The model under review builds one solid part; all positions refer to its coordinate system, in mm. Face numbers are marked on the shaded views. A direction names the side the tool comes from. Round coordinates to 2 decimals unless told otherwise and drop trailing zeros. Loops run counter-clockwise (first coordinate to the right, second up) from the corner with the lowest first, then second, coordinate; pieces in that order, holes last. Notation, with made-up numbers: (9.25, 53) -> (30.25, 53) arc R17 ccw to (30.25, 81) -> close; hole circle Ø8 at (51, 62.5). An arc over 180 degrees is marked (long way). Use CSV: the item, a comma, the result in double quotes. Start each with the question number.
```python
from build123d import *

# Parameters (mm, degrees)
SKETCH1_W           = 600
SKETCH1_H           = 310
BOSS_EXTRUDE1_DEPTH = 50
SKETCH2_W           = 515
SKETCH2_H           = 270
BOSS_EXTRUDE2_DEPTH = 160
SKETCH3_R           = 75
BOSS_EXTRUDE3_DEPTH = 26
SKETCH4_W           = 30
SKETCH4_H           = 12
BOSS_EXTRUDE4_DEPTH = 50


with BuildPart() as part:
    # Sketch1 → Boss-Extrude1 (new body)
    with BuildSketch(Plane(origin=(0, 0, 0), x_dir=(1, 0, 0), z_dir=(0, 1, 0))):
        Rectangle(SKETCH1_W, SKETCH1_H)
    extrude(amount=BOSS_EXTRUDE1_DEPTH)

    # Sketch2 → Boss-Extrude2 (add)
    with BuildSketch(Plane(origin=(0, 50, 0), x_dir=(1, 0, 0), z_dir=(0, 1, 0))):
        with Locations((0, 20)):
            Rectangle(SKETCH2_W, SKETCH2_H)
    extrude(amount=BOSS_EXTRUDE2_DEPTH)

    # Sketch3 → Boss-Extrude3 (add)
    with BuildSketch(Plane(origin=(0, 210, 0), x_dir=(1, 0, 0), z_dir=(0, 1, 0))):
        with Locations((0, 65)):
            Circle(SKETCH3_R)
    extrude(amount=BOSS_EXTRUDE3_DEPTH)

    # Sketch4 → Boss-Extrude4 (add)
    with BuildSketch(Plane(origin=(147.5, 0, 0), x_dir=(0, 0, -1), z_dir=(1, 0, 0))):
        with Locations((-65, 216)):
            Rectangle(SKETCH4_W, SKETCH4_H)
    extrude(amount=-BOSS_EXTRUDE4_DEPTH)


solid = part.part
```
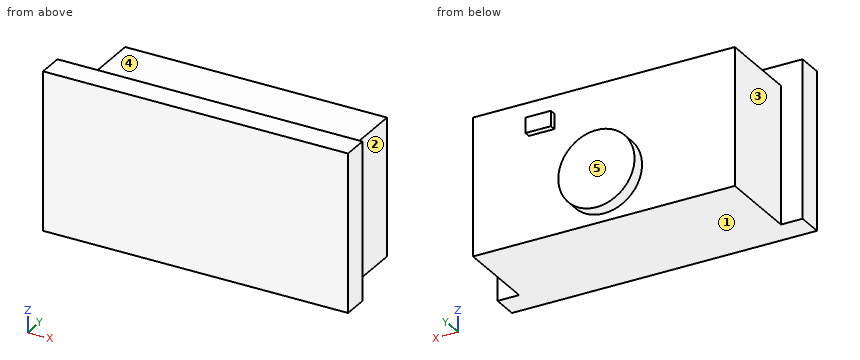
1. For the marked faces 1, 2, 3, 4 and 5, list the 3-axis set-ups (+Z, -Z, +X, -X, +Y, -Y) from which the entire face can be reached by the end or side of a thin tool; tool diameter is ignored.
2. Take a section at B-B, the plane x = 0. Give the boundary of the cut face in (y, z), then the cut area to 3 significant figures.
3. Clearance check with flat-ended pins moving along their axes: P1, Ø9.5, axis at y = 214.5, z = 65.5, coming from the +X side; P2, Ø13, axis at y = 215.5, z = 61.5, coming from the -X side; P3, Ø9.5, axis at x = 126, y = 215.5, coming from the +Z side. State where each tip first meets the part, or that it passes through.
4. Take a section at A-A, the plane z = 100. Give the boundary of the cut face in (x, y).
5. Take a section at D-D, the plane z = -65. Give the boundary of the cut face in (x, y), then the cut area to 3 significant figures.
6. Take a section at C-C, the plane y = 98. Give the boundary of the cut face in (x, z), then the cut area to 3 significant figures.
7. For line 1 along Y through (x, z) = (-180, -104.5); line 2 along X through (y, z) = (89, -51.5); line 3 along Y through (x, z) = (3.5, 116.5), list the stretches that pass through material, from the lowest coordinate up. Write a range as from..to.
Results:
1,face 1,"-Z, +X, -X, +Y, -Y"
1,face 2,"+Z, -Z, +X, +Y"
1,face 3,"+Z, -Z, -X, +Y"
1,face 4,"+Z, +X, -X, +Y"
1,face 5,"+Z, -Z, +X, -X, +Y"
2,outline,"(0, -155) -> (210, -155) -> (210, -140) -> (236, -140) -> (236, 10) -> (210, 10) -> (210, 115) -> (50, 115) -> (50, 155) -> (0, 155) -> close"
2,area,"62,600 mm²"
3,P1,"x = 257.5"
3,P2,"x = -257.5"
3,P3,"z = 80"
4,outline,"(-300, 0) -> (300, 0) -> (300, 50) -> (257.5, 50) -> (257.5, 210) -> (-257.5, 210) -> (-257.5, 50) -> (-300, 50) -> close"
5,outline,"(-300, 0) -> (300, 0) -> (300, 50) -> (257.5, 50) -> (257.5, 210) -> (75, 210) -> (75, 236) -> (-75, 236) -> (-75, 210) -> (-257.5, 210) -> (-257.5, 50) -> (-300, 50) -> close"
5,area,"116,000 mm²"
6,outline,"(-257.5, -155) -> (257.5, -155) -> (257.5, 115) -> (-257.5, 115) -> close"
6,area,"139,000 mm²"
7,line 1,"0..210"
7,line 2,"-257.5..257.5"
7,line 3,"0..50"
